Can you work these out from the drawing? Everything is in mm from the part's minimum corner. Coordinates: 2 decimals unless noted, no trailing zeros. Answer as CSV lines item,"result". Start each with the question number.
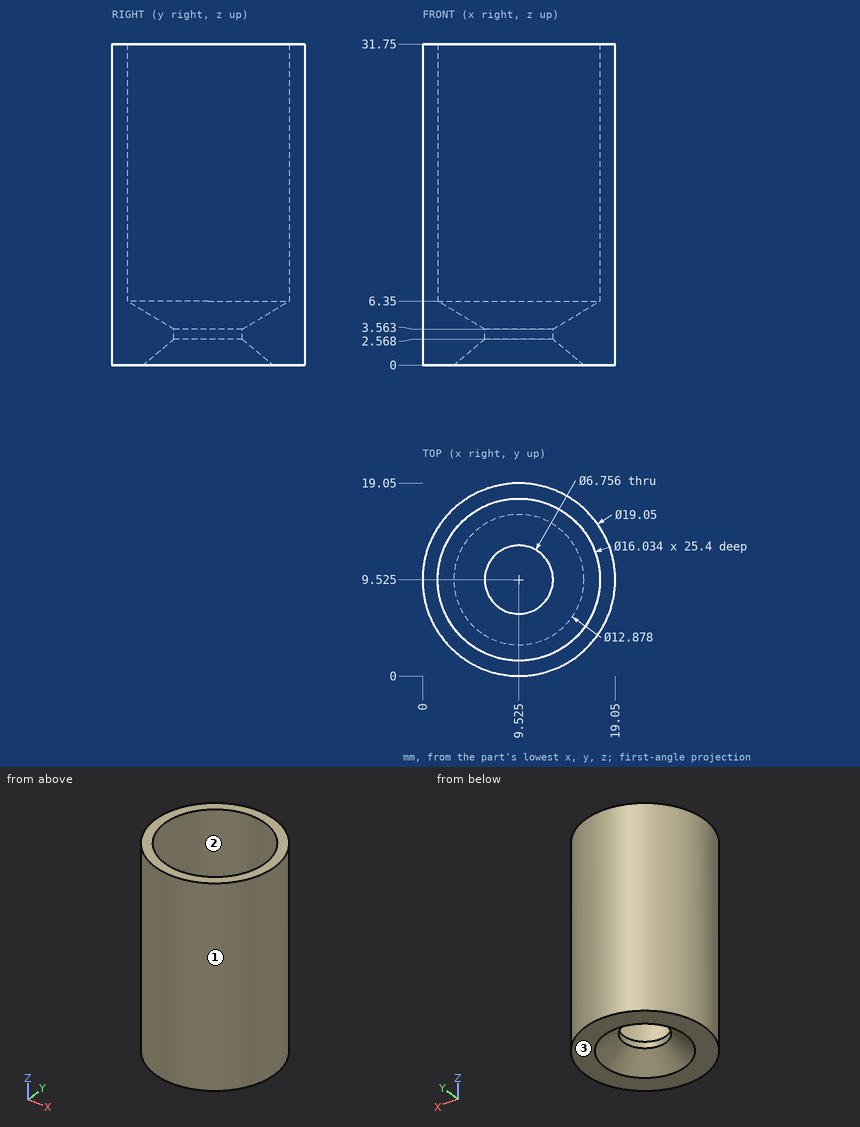
1) I need wall thicknesses on line 1 (Y direction, x = 9.5, z = 8); line 2 (Y direction, x = 15.5, z = 21.5) (1 decimal); line 3 (X direction, y = 11, z = 30) (1 decimal). Which ranges of each line are inside material? Lowest first, please. Write a range as [from, to].
2) Will these pins go through, and if not, where does the flat tip stop? pin 1 Ø4 at (x, z) = (13, 19.5) entering from -Y (1 decimal); pin 2 Ø1 at (y, z) = (11, 19) entering from -X; pin 3 Ø8 at (x, y) = (9.525, 9.525) entering from +Z.
3) If we mould it in two halves opening along Y, with no side actions, what happens to the marked faces 1, 2 and 3? For each: released by +Y, released by -Y, zero draft, split by the parting line, or undercut.
Output:
1,line 1,"[0, 1.51], [17.54, 19.05]"
1,line 2,"[2.1, 4.2], [14.9, 16.9]"
1,line 3,"[0.1, 1.6], [17.4, 18.9]"
2,pin 1,"y = 0.1"
2,pin 2,"x = 0.05"
2,pin 3,"z = 3.94"
3,face 1,"split by the parting line"
3,face 2,"undercut"
3,face 3,"zero draft"
